from build123d import *

# Parameters (mm, degrees)
F0_R     = 19
F1_DEPTH = 5
F4_D     = 5.5
F6_D     = 6


# Not quite as in the source:
# - a feature names something its author has since deleted; it is built from what else it names


with BuildPart() as f1:
    # F0 (on Front) → F1 (new body)
    with BuildSketch(Plane.XZ):
        Circle(F0_R)
    extrude(amount=F1_DEPTH)

    # F4 (through all)
    with Locations(Plane.XZ.offset(5)):
        with Locations((-6.9282032303, -4), (0, 8), (6.9282032303, -4)):
            Hole(F4_D / 2)

    # F6 (through all)
    with Locations(Plane.XZ.offset(5)):
        with Locations((0, 0)):
            Hole(F6_D / 2)


solid = f1.part
Verification items for the finished model (mm, model axes). Coordinates: 2 decimals unless noted, no trailing zeros. Order: outer loops, then holes, each group sorted by start corner. A loop starts at its lowest first (then second) coordinate and runs counter-clockwise, first axis right, second up. Notation, with made-up numbers: (25, 82) -> (30, 82) arc R15 cw to (30, 87) -> close; hole circle Ø2 at (33.5, 24.5). An arc over 180 degrees is marked (long way). Put each result on its own line as item: value. Start each with the question number.
1. Cross-section at B-B, the plane z = 0. Record the boundary of the cut face in (x, y).
2. Cross-section at C-C, the plane z = -4. Record the boundary of the cut face in (x, y), then the cut area to 3 significant figures.
3. Cross-section at D-D, the plane y = -3.9. Record the boundary of the cut face in (x, z).
4. Cross-section at A-A, the plane x = 0. Record the boundary of the cut face in (y, z), then the cut area to 4 significant figures.
5. Mould release check, pull along X, two halves, no side actions. Record for faces 1 (the cylindrical face through (0.596, -2.465, 5.315)), 2 (the cylindrical face through (8.767, -2.465, -16.856)), 3 (the flat face through (4, -5, 0)): released by +X, released by -X, zero draft, split by the parting line, or undercut.
6. Go/stop test with flat-tipped pins: pin 1 Ø3.5 at (x, z) = (-6.93, -4) entering from +Y; pin 2 Ø1 at (x, y) = (3.5, -3) entering from +Z; pin 3 Ø1 at (y, z) = (-3, 5) entering from +X. Record where each tip stops, or that it passes through.
7. Material ranges on L1, parallel to Z at x = -2, y = -4.15; L2, parallel to X at y = -4.25, z = 1.5; L3, parallel to Z at x = -0.5, y = -0.85, recorded low to high. Write a range as [from, to].
Computed:
1. outline: (-19, -5) -> (-3, -5) -> (-3, 0) -> (-19, 0) -> close; (3, -5) -> (19, -5) -> (19, 0) -> (3, 0) -> close
2. outline: (-18.57, -5) -> (-9.68, -5) -> (-9.68, 0) -> (-18.57, 0) -> close; (-4.18, -5) -> (4.18, -5) -> (4.18, 0) -> (-4.18, 0) -> close; (9.68, -5) -> (18.57, -5) -> (18.57, 0) -> (9.68, 0) -> close
2. area: 131 mm2
3. outline: circle Ø38 at (0, 0); hole circle Ø5.5 at (-6.93, -4); hole circle Ø6 at (0, 0); hole circle Ø5.5 at (0, 8); hole circle Ø5.5 at (6.93, -4)
4. outline: (-5, -19) -> (0, -19) -> (0, -3) -> (-5, -3) -> close; (-5, 3) -> (0, 3) -> (0, 5.25) -> (-5, 5.25) -> close; (-5, 10.75) -> (0, 10.75) -> (0, 19) -> (-5, 19) -> close
4. area: 132.5 mm2
5. face 1: undercut
5. face 2: split by the parting line
5. face 3: zero draft
6. pin 1: through
6. pin 2: z = 18.76
6. pin 3: x = 18.46
7. L1: [-18.89, -2.24], [2.24, 6.11], [9.89, 18.89]
7. L2: [-18.94, -2.6], [2.6, 18.94]
7. L3: [-18.99, -2.96], [2.96, 5.3], [10.7, 18.99]
